```python
from build123d import *

# Parameters (mm, degrees)
SCHIZZO1_W                                           = 80
SCHIZZO1_H                                           = 18
ESTRUSIONE_ESTRUSIONE1_DEPTH                         = 45
SMUSSO1_SIZE                                         = 3.8
SMUSSO1_SIZE2                                        = 6.581793069
SMUSSO2_SIZE                                         = 3.8
SMUSSO2_SIZE2                                        = 6.581793069
SCHIZZO2_W                                           = 9.6
SCHIZZO2_H                                           = 13.6
ESTRUSIONE_ESTRUSIONE2_DEPTH                         = 50
SMUSSO3_SIZE                                         = 1.5
FORO_PER_VITE_M4_1_D                                 = 5.6
FORO_PER_VITE_M4_1_DEPTH                             = 50
FORO_PER_VITE_M4_1_TIP                               = 1.682409733
FORO_LAMATO_PER_BULLONE_M5_A_TESTA_ESAGO_D           = 5.6
FORO_LAMATO_PER_BULLONE_M5_A_TESTA_ESAGO_DEPTH       = 50
FORO_LAMATO_PER_BULLONE_M5_A_TESTA_ESAGO_CBORE_D     = 13
FORO_LAMATO_PER_BULLONE_M5_A_TESTA_ESAGO_CBORE_DEPTH = 3
FORO_LAMATO_PER_BULLONE_M5_A_TESTA_ESAGO_TIP         = 1.682409733
FORO_LAMATO_PER_BULLONE_M5_A_TESTA_E_2_D             = 5.6
FORO_LAMATO_PER_BULLONE_M5_A_TESTA_E_2_DEPTH         = 50
FORO_LAMATO_PER_BULLONE_M5_A_TESTA_E_2_CBORE_D       = 13
FORO_LAMATO_PER_BULLONE_M5_A_TESTA_E_2_CBORE_DEPTH   = 3
FORO_LAMATO_PER_BULLONE_M5_A_TESTA_E_2_TIP           = 1.682409733


with BuildPart() as part:
    # Schizzo1 → Estrusione-Estrusione1 (new body)
    with BuildSketch(Plane.XY):
        with Locations((-40, 9)):
            Rectangle(SCHIZZO1_W, SCHIZZO1_H)
    extrude(amount=ESTRUSIONE_ESTRUSIONE1_DEPTH)

    # Smusso1
    smusso1_edges = [part.edges().sort_by_distance(p)[0] for p in [
        (0, 18, 22.5),
    ]]
    smusso1_side = [part.faces().sort_by_distance(p)[0] for p in [
        (0, 9, 22.5),
    ]]
    chamfer(smusso1_edges, length=SMUSSO1_SIZE, length2=SMUSSO1_SIZE2, reference=smusso1_side[0])

    # Smusso2
    smusso2_edges = [part.edges().sort_by_distance(p)[0] for p in [
        (0, 0, 22.5),
    ]]
    smusso2_side = [part.faces().sort_by_distance(p)[0] for p in [
        (0, 7.1, 22.5),
    ]]
    chamfer(smusso2_edges, length=SMUSSO2_SIZE, length2=SMUSSO2_SIZE2, reference=smusso2_side[0])

    # Schizzo2 → Estrusione-Estrusione2 (add)
    with BuildSketch(Plane.ZY.offset(80)):
        with Locations((5, 9)):
            Rectangle(SCHIZZO2_W, SCHIZZO2_H)
        with Locations((40, 9)):
            Rectangle(SCHIZZO2_W, SCHIZZO2_H)
    extrude(amount=ESTRUSIONE_ESTRUSIONE2_DEPTH)

    # Smusso3
    smusso3_edges = [part.edges().sort_by_distance(p)[0] for p in [
        (-105, 15.8, 0.2),
        (-105, 2.2, 0.2),
        (-105, 2.2, 9.8),
        (-105, 15.8, 9.8),
        (-130, 9, 0.2),
        (-130, 2.2, 5),
        (-130, 9, 9.8),
        (-130, 15.8, 5),
        (-105, 15.8, 35.2),
        (-105, 2.2, 35.2),
        (-105, 2.2, 44.8),
        (-105, 15.8, 44.8),
        (-130, 9, 35.2),
        (-130, 2.2, 40),
        (-130, 9, 44.8),
        (-130, 15.8, 40),
    ]]
    chamfer(smusso3_edges, length=SMUSSO3_SIZE)

    # Foro per Vite M4-1
    with Locations(Plane(origin=(-115, 9, 0.2), x_dir=(0, -1, 0), z_dir=(0, 0, -1))):
        with Locations((0, 0), (0, -20)):
            Hole(FORO_PER_VITE_M4_1_D / 2, depth=FORO_PER_VITE_M4_1_DEPTH)
            with Locations((0, 0, -(FORO_PER_VITE_M4_1_DEPTH + FORO_PER_VITE_M4_1_TIP / 2))):  # 118° drill point
                Cone(0, FORO_PER_VITE_M4_1_D / 2, FORO_PER_VITE_M4_1_TIP, mode=Mode.SUBTRACT)

    # Foro lamato per Bullone M5 a testa esago
    with Locations(Plane.XY.offset(45)):
        with Locations((-9, 9), (-55, 9)):
            CounterBoreHole(FORO_LAMATO_PER_BULLONE_M5_A_TESTA_ESAGO_D / 2, FORO_LAMATO_PER_BULLONE_M5_A_TESTA_ESAGO_CBORE_D / 2, FORO_LAMATO_PER_BULLONE_M5_A_TESTA_ESAGO_CBORE_DEPTH, depth=FORO_LAMATO_PER_BULLONE_M5_A_TESTA_ESAGO_DEPTH)
            with Locations((0, 0, -(FORO_LAMATO_PER_BULLONE_M5_A_TESTA_ESAGO_DEPTH + FORO_LAMATO_PER_BULLONE_M5_A_TESTA_ESAGO_TIP / 2))):  # 118° drill point
                Cone(0, FORO_LAMATO_PER_BULLONE_M5_A_TESTA_ESAGO_D / 2, FORO_LAMATO_PER_BULLONE_M5_A_TESTA_ESAGO_TIP, mode=Mode.SUBTRACT)

    # Foro lamato per Bullone M5 a testa e 2
    with Locations(Plane(origin=(-9, 9, 0), x_dir=(-1, 0, 0), z_dir=(0, 0, -1))):
        with Locations((0, 0), (46, 0)):
            CounterBoreHole(FORO_LAMATO_PER_BULLONE_M5_A_TESTA_E_2_D / 2, FORO_LAMATO_PER_BULLONE_M5_A_TESTA_E_2_CBORE_D / 2, FORO_LAMATO_PER_BULLONE_M5_A_TESTA_E_2_CBORE_DEPTH, depth=FORO_LAMATO_PER_BULLONE_M5_A_TESTA_E_2_DEPTH)
            with Locations((0, 0, -(FORO_LAMATO_PER_BULLONE_M5_A_TESTA_E_2_DEPTH + FORO_LAMATO_PER_BULLONE_M5_A_TESTA_E_2_TIP / 2))):  # 118° drill point
                Cone(0, FORO_LAMATO_PER_BULLONE_M5_A_TESTA_E_2_D / 2, FORO_LAMATO_PER_BULLONE_M5_A_TESTA_E_2_TIP, mode=Mode.SUBTRACT)


solid = part.part
```
Model file for the job. Use its own axes, mm. A direction names the side the tool comes from. Coordinates: 2 decimals unless noted, no trailing zeros. Loops run counter-clockwise (first coordinate to the right, second up) from the corner with the lowest first, then second, coordinate; pieces in that order, holes last. Notation, with made-up numbers: (54, -9.5) -> (76, -9.5) arc R20 ccw to (76, 10.5) -> close; hole circle Ø10 at (36, -22.75). An arc over 180 degrees is marked (long way). Answer as a JSON object with one key per item and string values.
Q1. Cut at C-C (z = 38). List the corners of the cut face in (x, y).
Report:
{"outline": "(-130, 3.7) -> (-128.5, 2.2) -> (-80, 2.2) -> (-80, 0) -> (-6.58, 0) -> (0, 3.8) -> (0, 14.2) -> (-6.58, 18) -> (-80, 18) -> (-80, 15.8) -> (-128.5, 15.8) -> (-130, 14.3) -> close; hole circle Ø5.6 at (-115, 9); hole circle Ø5.6 at (-95, 9); hole circle Ø5.6 at (-55, 9); hole circle Ø5.6 at (-9, 9)"}
Q2. 3-axis set-ups, long thin cutter, end or side, ignore diameter. For faces 1 (the cylindrical face through (-2.8, 10.95, 43.52)), 2 (the flat face through (-104, 15.8, 5)), 3 (the flat face through (-104, 2.2, 5)), 4 (the flat face through (-12, 8, 3)): which of +Z, -Z, +X, -X, +Y, -Y reach the whole face in a straight line?
Report:
{"face 1": "+Z", "face 2": "+Z, -Z, -X, +Y", "face 3": "+Z, -Z, -X, -Y", "face 4": "-Z"}
Q3. Pull direction Y, two halves, no side cores. Call faces 5 (the flat face through (-44, 0, 22)), 6 (the flat face through (-41, 9, 0)), 7 (the cylindrical face through (-61.2, 10.95, 1.48)): released by +Y, released by -Y, zero draft, split by the parting line, or undercut.
Report:
{"face 5": "released by -Y", "face 6": "zero draft", "face 7": "undercut"}
Q4. Probe probe 1 along X at (y, z) = (9, 41); probe 2 along X at (y, z) = (9, 24); probe 3 along X at (y, z) = (11.5, 7). List the from-to ranges inside material, lowest first.
Report:
{"probe 1": "x = -130 to -117.8, -112.2 to -97.8, -92.2 to -57.8, -52.2 to -11.8, -6.2 to 0", "probe 2": "x = -80 to -57.8, -52.2 to -11.8, -6.2 to 0", "probe 3": "x = -130 to -116.26, -113.74 to -96.26, -93.74 to -56.26, -53.74 to -10.26, -7.74 to 0"}
Q5. Cut at D-D (y = 9). State how many separate pieces and enclosed holes the cut face has, and give its area (3 significant figures).
Report:
{"separate pieces": "7", "enclosed holes": "0", "area": "3,750 mm2"}
Q6. Flat gauge pins, fed straight in: P1, Ø10, axis at y = 5.5, z = 24.5, coming from the -X side; P2, Ø8, axis at x = -55, y = 9, coming from the -Z side; P3, Ø4.5, axis at x = -115, y = 9, coming from the +Z side; P4, Ø5.5, axis at x = -99, z = 6.5, coming from the -Y side. Where does each tip first touch, or does it go through?
Report:
{"P1": "stops at x = -80", "P2": "stops at z = 3", "P3": "passes through", "P4": "stops at y = 2.2"}
Q7. Cut at B-B (z = 17.5). List the corners of the cut face in (x, y).
Report:
{"outline": "(-80, 0) -> (-6.58, 0) -> (0, 3.8) -> (0, 14.2) -> (-6.58, 18) -> (-80, 18) -> close; hole circle Ø5.6 at (-55, 9); hole circle Ø5.6 at (-9, 9)"}
Q8. Cut at A-A (x = -83.5). List the corners of the cut face in (y, z), and give its area (3 significant figures).
Report:
{"outline": "(2.2, 1.7) -> (3.7, 0.2) -> (14.3, 0.2) -> (15.8, 1.7) -> (15.8, 8.3) -> (14.3, 9.8) -> (3.7, 9.8) -> (2.2, 8.3) -> close; (2.2, 36.7) -> (3.7, 35.2) -> (14.3, 35.2) -> (15.8, 36.7) -> (15.8, 43.3) -> (14.3, 44.8) -> (3.7, 44.8) -> (2.2, 43.3) -> close", "area": "252 mm2"}
